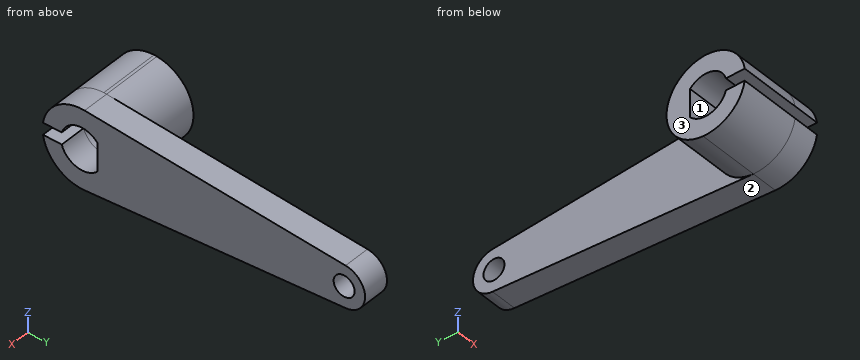
from build123d import *

# Parameters (mm, degrees)
BOSS_EXTRUDE1_DEPTH      = 2.5
BOSS_EXTRUDE1_DEPTH_BACK = 2.5
SKETCH2_R                = 2
CUT_EXTRUDE1_REACH       = 56.747
SKETCH3_W                = 2.263959938
SKETCH3_H                = 7.327028906
BOSS_EXTRUDE2_START      = 11.5
BOSS_EXTRUDE2_DEPTH      = 11.5


with BuildPart() as part:
    # Sketch2 → Boss-Extrude1 (new, two sides: drawn at the far end of the back side and taken through both)
    with BuildSketch(Plane(origin=(0, 0, 0), x_dir=(0, 0, -1), z_dir=(1, 0, 0)).offset(-BOSS_EXTRUDE1_DEPTH_BACK)):
        with BuildLine():
            Line((3.990187965, 50.28), (7.481602435, 0.525))
            ThreePointArc((7.481602435, 0.525), (0, -7.5), (-7.481602435, 0.525))
            Line((-7.481602435, 0.525), (-3.990187965, 50.28))
            ThreePointArc((-3.990187965, 50.28), (0, 54), (3.990187965, 50.28))
        make_face()
        with Locations((0, 50)):
            Circle(SKETCH2_R, mode=Mode.SUBTRACT)
        with BuildLine():
            ThreePointArc((-2.645751311, 3), (0, -4), (2.645751311, 3))
            Line((2.645751311, 3), (-2.645751311, 3))
        make_face(mode=Mode.SUBTRACT)
    extrude(amount=BOSS_EXTRUDE1_DEPTH + BOSS_EXTRUDE1_DEPTH_BACK)

    # Sketch3 → Cut-Extrude1 (cut, up to next)
    with BuildSketch(Plane(origin=(2.5, 0, 0), x_dir=(0, 0, -1), z_dir=(1, 0, 0)), mode=Mode.PRIVATE) as cut_extrude1_sk1:
        with Locations((0, -7.5)):
            Rectangle(SKETCH3_W, SKETCH3_H)
    cut_extrude1_tool1 = extrude(cut_extrude1_sk1.sketch, amount=-CUT_EXTRUDE1_REACH, mode=Mode.PRIVATE) & part.part
    add(cut_extrude1_tool1.solids().sort_by_distance((2.5, -7.5, 0))[0], mode=Mode.SUBTRACT)

    # Sketch5 → Boss-Extrude2 (add)
    with BuildSketch(Plane.ZY.offset(2.5).offset(BOSS_EXTRUDE2_START)):
        with BuildLine():
            ThreePointArc((-7.481602435, 0.525), (-5.85710754, -4.684473424), (-1.131979969, -7.414082637))
            Line((-1.131979969, -7.414082637), (-1.131979969, -3.836485547))
            ThreePointArc((-1.131979969, -3.836485547), (-3.905406133, -0.864755998), (-2.645751311, 3))
            Line((-2.645751311, 3), (2.645751311, 3))
            ThreePointArc((2.645751311, 3), (3.905406133, -0.864755998), (1.131979969, -3.836485547))
            Line((1.131979969, -3.836485547), (1.131979969, -7.414082637))
            ThreePointArc((1.131979969, -7.414082637), (5.689457345, -4.886724375), (7.5, 0))
            ThreePointArc((7.5, 0), (7.495399198, 0.262661127), (7.481602435, 0.525))
            ThreePointArc((7.481602435, 0.525), (0, 7.5), (-7.481602435, 0.525))
        make_face()
    extrude(amount=-BOSS_EXTRUDE2_DEPTH)


solid = part.part
Geometry check sheet. Reference: the model listing, model coordinates, mm. Face numbers are marked on the shaded views. Give positions to 0.01 mm unless a question says otherwise; leave off trailing zeros. Order: outer loops, then holes, each group sorted by start corner. A loop starts at its lowest first (then second) coordinate and runs counter-clockwise, first axis right, second up. Notation, with made-up numbers: M 48.5,-30 L 81.5,-30 A18 cw 81.5,-26 Z; hole C 30.5,-26.5 d11. An arc over 180 degrees is marked long. Use a Markdown table: item, result.
Item 1: Section check D-D (z = 3.25). Record the cut outline in (x, y).
Answers follow:
| item | result |
|---|---|
| outline | M -14,-6.76 L 2.5,-6.76 L 2.5,-2.33 L -14,-2.33 Z; M -14,2.33 L 2.5,2.33 L 2.5,52.33 L -2.5,52.33 L -2.5,6.76 L -14,6.76 Z |
Item 2: Material ranges on line 1 along Y through (x, z) = (0.35, 0); line 2 along X through (y, z) = (34, 2); line 3 along Z through (x, y) = (-12, -2.5), recorded low to high.
Answers follow:
| item | result |
|---|---|
| line 1 | y = 3 to 48, 52 to 54 |
| line 2 | x = -2.5 to 2.5 |
| line 3 | z = -7.07 to -3.12, 3.12 to 7.07 |
Item 3: Depth check by flat-ended pin: P1, Ø6, axis at x = -6, z = 0.5, coming from the -Y side; P2, Ø1, axis at x = -1.5, y = 35, coming from the -Z side; P3, Ø1.1, axis at x = -4.5, y = -5, coming from the -Z side. Enter the tip coordinate at first touch or a pass-through.
Answers follow:
| item | result |
|---|---|
| P1 | stops at y = -7.41 |
| P2 | stops at z = -5.1 |
| P3 | stops at z = -6.04 |
Item 4: Section check C-C (x = -9.5). Record the cut outline in (y, z) (3 decimals), and give its area (3 significant figures).
Answers follow:
| item | result |
|---|---|
| outline | M -7.414,-1.132 A7.5 ccw long -7.414,1.132 L -3.836,1.132 A4 cw 3,2.646 L 3,-2.646 A4 cw -3.836,-1.132 Z |
| area | 122 mm2 |
Item 5: Section check A-A (z = 0). Record the cut outline in (x, y), and give its area (3 significant figures).
Answers follow:
| item | result |
|---|---|
| outline | M -14,3 L 2.5,3 L 2.5,48 L -2.5,48 L -2.5,7.5 L -14,7.5 Z; M -2.5,52 L 2.5,52 L 2.5,54 L -2.5,54 Z |
| area | 287 mm2 |
Item 6: Draft check along Z on the marked faces 1, 2 and 3. Enter one of: +Z half, -Z half, draft (parallel to the pull), parting line (faces both ways), or undercut.
Answers follow:
| item | result |
|---|---|
| face 1 | undercut |
| face 2 | -Z half |
| face 3 | draft |
Item 7: Section check B-B (x = 0). Record the cut outline in (y, z) (3 decimals), and give its area (3 significant figures).
Answers follow:
| item | result |
|---|---|
| outline | M -7.414,-1.132 A7.5 ccw 0.525,-7.482 L 50.28,-3.99 A4 ccw 50.28,3.99 L 0.525,7.482 A7.5 ccw -7.414,1.132 L -3.836,1.132 A4 cw 3,2.646 L 3,-2.646 A4 cw -3.836,-1.132 Z; hole C 50,0 d4 |
| area | 623 mm2 |
